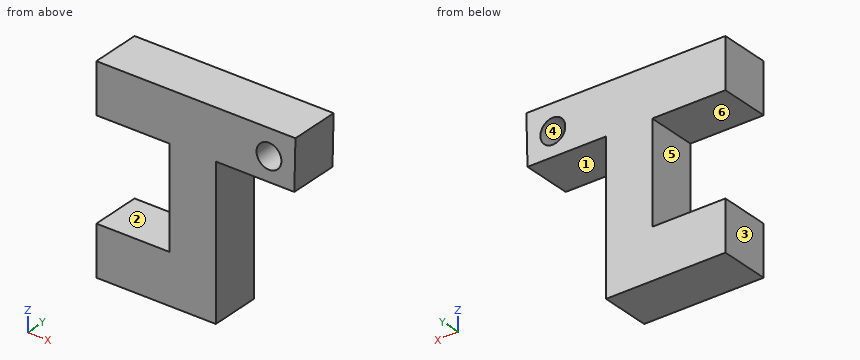
```python
from build123d import *

# Parameters (mm, degrees)
F0_W     = 25.4
F0_H     = 25.4
F1_DEPTH = 6.35
F2_W     = 9.33873
F2_H     = 12.7
F3_DEPTH = 25.4
F4_R     = 1.5875
F5_DEPTH = 25.4


with BuildPart() as f1:
    # F0 (on Front) → F1 (new body)
    with BuildSketch(Plane.XZ):
        with Locations((12.7, 12.7)):
            Rectangle(F0_W, F0_H)
    extrude(amount=F1_DEPTH)

    # F2 (on face) → F3 (cut)
    with BuildSketch(Plane.XZ.offset(6.35)):
        with Locations((4.669365, 12.7)):
            Rectangle(F2_W, F2_H)
        Polygon((25.4, 0), (25.4, 25.4), (25.255403, 19.05), (15.24, 19.05), (15.24, 0), align=None)
    extrude(amount=-F3_DEPTH, mode=Mode.SUBTRACT)

    # F4 (on face) → F5 (cut)
    with BuildSketch(Plane.XZ.offset(6.35)):
        with Locations((22.022767, 22.086186)):
            Circle(F4_R)
    extrude(amount=-F5_DEPTH, mode=Mode.SUBTRACT)


solid = f1.part
```
For this review, take the finished solid that the model builds, in its own axes (mm). Face numbers are marked on the shaded views. A direction names the side the tool comes from. Coordinates: 2 decimals unless noted, no trailing zeros. Order: outer loops, then holes, each group sorted by start corner. A loop starts at its lowest first (then second) coordinate and runs counter-clockwise, first axis right, second up. Notation, with made-up numbers: (23.25, 50) -> (32.25, 50) arc R20 cw to (32.25, 82) -> close; hole circle Ø2 at (27.25, -11.75). An arc over 180 degrees is marked (long way). Use CSV: the item, a comma, the result in double quotes. Start each with the question number.
Item 1: We need section D-D, the plane z = 11.5. Give the boundary of the cut face in (x, y).
Item 2: Draft analysis for pull direction X (two halves, no side actions). For the marked faces 4, 5 and 6, state which applies: pulls with the +X half, pulls with the -X half, needs draft (parallel to the pull), parting line crosses it, or undercut.
Item 3: Insertion check: pin 1 (3 mm diameter, centred on y = -1, z = 8.5, fed in from +X); pin 2 (3 mm diameter, centred on y = -2, z = 11, fed in from -X); pin 3 (1.5 mm diameter, centred on x = 10, z = 14, fed in from +Y); pin 4 (3 mm diameter, centred on x = 18.5, y = -3.5, fed in from -Z). Each pin has a flat end and moves straight along its axis. Give the tip position at first contact, or say it passes through.
Item 4: We need section A-A, the plane z = 22.5. Give the boundary of the cut face in (x, y).
Item 5: Wall thickness on probe 1 along Z at (x, y) = (2, -2.25); probe 2 along Z at (x, y) = (22, -0.75); probe 3 along X at (y, z) = (-5, 1.5): over which ranges is each line inside the solid? List them lowest first.
Item 6: We need section C-C, the plane x = 16. Give the boundary of the cut face in (y, z), then the cut area to 3 significant figures.
Item 7: For the marked faces 1, 2 and 3, list the 3-axis set-ups (+Z, -Z, +X, -X, +Y, -Y) from which the entire face can be reached by the end or side of a thin tool; tool diameter is ignored.
Derived:
1,outline,"(9.34, -6.35) -> (15.24, -6.35) -> (15.24, 0) -> (9.34, 0) -> close"
2,face 4,"undercut"
2,face 5,"pulls with the -X half"
2,face 6,"needs draft"
3,pin 1,"stops at x = 15.24"
3,pin 2,"stops at x = 9.34"
3,pin 3,"stops at y = 0"
3,pin 4,"stops at z = 19.05"
4,outline,"(0, -6.35) -> (20.49, -6.35) -> (20.49, 0) -> (0, 0) -> close; (23.56, -6.35) -> (25.33, -6.35) -> (25.33, 0) -> (23.56, 0) -> close"
5,probe 1,"z = 0 to 6.35, 19.05 to 25.4"
5,probe 2,"z = 19.05 to 20.5, 23.67 to 25.4"
5,probe 3,"x = 0 to 15.24"
6,outline,"(-6.35, 19.05) -> (0, 19.05) -> (0, 25.4) -> (-6.35, 25.4) -> close"
6,area,"40.3 mm^2"
7,face 1,"-Z, +X, +Y, -Y"
7,face 2,"-X, +Y, -Y"
7,face 3,"+Z, -Z, -X, +Y, -Y"
